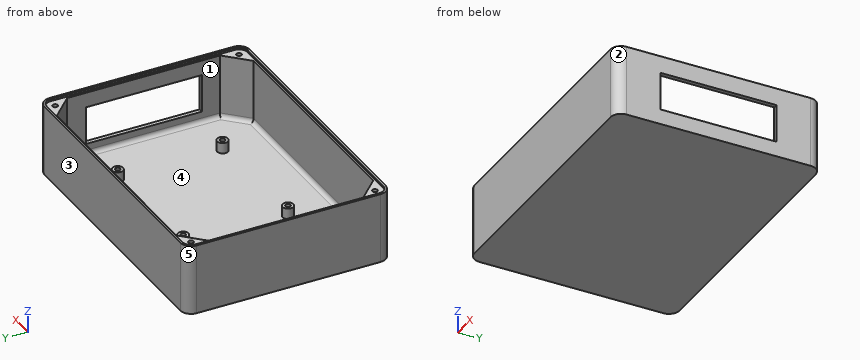
from build123d import *

# Parameters (mm, degrees)
BOSS_EXTRUDE1_DEPTH = 2
BOSS_EXTRUDE2_START = 30
SKETCH2_R           = 3
BOSS_EXTRUDE2_DEPTH = 30
SKETCH3_R           = 1.2
CUT_EXTRUDE1_DEPTH  = 25
BOSS_EXTRUDE3_START = 1
BOSS_EXTRUDE3_DEPTH = 1
SKETCH6_W           = 17.83
SKETCH6_H           = 54.204820934
CUT_EXTRUDE2_DEPTH  = 2
SKETCH7_R           = 2.5
SKETCH7_R_2         = 1.375
SKETCH7_R_3         = 1.2
BOSS_EXTRUDE4_DEPTH = 5
FILLET1_R           = 2


with BuildPart() as part:
    # Sketch1 → Boss-Extrude1 (new body)
    with BuildSketch(Plane(origin=(0, 0, -5), x_dir=(-1, 0, 0), z_dir=(0, 0, -1))):
        with BuildLine():
            Line((77.100439502, -47.051685991), (197.59949644, -47.051685991))
            ThreePointArc((197.59949644, -47.051685991), (201.135030346, -45.587219897), (202.59949644, -42.051685991))
            Line((202.59949644, -42.051685991), (202.59949644, 43.948314009))
            ThreePointArc((202.59949644, 43.948314009), (201.135030346, 47.483847915), (197.59949644, 48.948314009))
            Line((197.59949644, 48.948314009), (77.100439502, 48.948314009))
            ThreePointArc((77.100439502, 48.948314009), (73.564905596, 47.483847915), (72.100439502, 43.948314009))
            Line((72.100439502, 43.948314009), (72.100439502, -42.051685991))
            ThreePointArc((72.100439502, -42.051685991), (73.564905596, -45.587219897), (77.100439502, -47.051685991))
        make_face()
    extrude(amount=BOSS_EXTRUDE1_DEPTH)

    # Sketch2 → Boss-Extrude2 (add)
    # profile 1 of 7: a face of its own
    with BuildSketch(Plane.XY.offset(-5).offset(BOSS_EXTRUDE2_START)):
        with BuildLine():
            ThreePointArc((-202.59949644, -42.051685991), (-201.135030346, -45.587219897), (-197.59949644, -47.051685991))
            Line((-197.59949644, -47.051685991), (-77.100439502, -47.051685991))
            ThreePointArc((-77.100439502, -47.051685991), (-73.564905596, -45.587219897), (-72.100439502, -42.051685991))
            Line((-72.100439502, -42.051685991), (-72.100439502, 43.948314009))
            ThreePointArc((-72.100439502, 43.948314009), (-73.564905596, 47.483847915), (-77.100439502, 48.948314009))
            Line((-77.100439502, 48.948314009), (-197.59949644, 48.948314009))
            ThreePointArc((-197.59949644, 48.948314009), (-201.135030346, 47.483847915), (-202.59949644, 43.948314009))
            Line((-202.59949644, 43.948314009), (-202.59949644, -42.051685991))
        make_face()
        with BuildLine():
            Line((-74.100439502, -34.809045304), (-74.100439502, -42.051685991))
            ThreePointArc((-74.100439502, -42.051685991), (-74.979119158, -44.173006334), (-77.100439502, -45.051685991))
            Line((-77.100439502, -45.051685991), (-84.343080189, -45.051685991))
            Line((-84.343080189, -45.051685991), (-190.356855753, -45.051685991))
            Line((-190.356855753, -45.051685991), (-197.59949644, -45.051685991))
            ThreePointArc((-197.59949644, -45.051685991), (-199.720816783, -44.173006334), (-200.59949644, -42.051685991))
            Line((-200.59949644, -42.051685991), (-200.59949644, -34.809045304))
            Line((-200.59949644, -34.809045304), (-200.59949644, 36.705673322))
            Line((-200.59949644, 36.705673322), (-200.59949644, 43.948314009))
            ThreePointArc((-200.59949644, 43.948314009), (-199.720816783, 46.069634353), (-197.59949644, 46.948314009))
            Line((-197.59949644, 46.948314009), (-190.356855753, 46.948314009))
            Line((-190.356855753, 46.948314009), (-84.343080189, 46.948314009))
            Line((-84.343080189, 46.948314009), (-77.100439502, 46.948314009))
            ThreePointArc((-77.100439502, 46.948314009), (-74.979119158, 46.069634353), (-74.100439502, 43.948314009))
            Line((-74.100439502, 43.948314009), (-74.100439502, 36.705673322))
            Line((-74.100439502, 36.705673322), (-74.100439502, -34.809045304))
        make_face(mode=Mode.SUBTRACT)
    # profile 2 of 7: a face of its own
    with BuildSketch(Plane.XY.offset(-5).offset(BOSS_EXTRUDE2_START)):
        with BuildLine():
            Line((-197.59949644, -45.051685991), (-190.356855753, -45.051685991))
            Line((-190.356855753, -45.051685991), (-200.59949644, -34.809045304))
            Line((-200.59949644, -34.809045304), (-200.59949644, -42.051685991))
            ThreePointArc((-200.59949644, -42.051685991), (-199.720816783, -44.173006334), (-197.59949644, -45.051685991))
        make_face()
    # profile 3 of 7: a face of its own
    with BuildSketch(Plane.XY.offset(-5).offset(BOSS_EXTRUDE2_START)):
        with BuildLine():
            Line((-200.59949644, 36.705673322), (-190.356855753, 46.948314009))
            Line((-190.356855753, 46.948314009), (-197.59949644, 46.948314009))
            ThreePointArc((-197.59949644, 46.948314009), (-199.720816783, 46.069634353), (-200.59949644, 43.948314009))
            Line((-200.59949644, 43.948314009), (-200.59949644, 36.705673322))
        make_face()
    # profile 4 of 7: a face of its own
    with BuildSketch(Plane.XY.offset(-5).offset(BOSS_EXTRUDE2_START)):
        with BuildLine():
            Line((-84.343080189, 46.948314009), (-74.100439502, 36.705673322))
            Line((-74.100439502, 36.705673322), (-74.100439502, 43.948314009))
            ThreePointArc((-74.100439502, 43.948314009), (-74.979119158, 46.069634353), (-77.100439502, 46.948314009))
            Line((-77.100439502, 46.948314009), (-84.343080189, 46.948314009))
        make_face()
    # profile 5 of 7: a face of its own
    with BuildSketch(Plane.XY.offset(-5).offset(BOSS_EXTRUDE2_START)):
        with BuildLine():
            ThreePointArc((-79.221759818, -39.93036562), (-75.952389187, -39.280047401), (-74.100439502, -42.051685991))
            Line((-74.100439502, -42.051685991), (-74.100439502, -34.809045304))
            Line((-74.100439502, -34.809045304), (-79.221759818, -39.93036562))
        make_face()
    # profile 6 of 7: a face of its own
    with BuildSketch(Plane.XY.offset(-5).offset(BOSS_EXTRUDE2_START)):
        with Locations((-77.100439502, -42.051685991)):
            Circle(SKETCH2_R)
    # profile 7 of 7: a face of its own
    with BuildSketch(Plane.XY.offset(-5).offset(BOSS_EXTRUDE2_START)):
        with BuildLine():
            Line((-84.343080189, -45.051685991), (-77.100439502, -45.051685991))
            ThreePointArc((-77.100439502, -45.051685991), (-79.872078107, -43.19973627), (-79.221759818, -39.93036562))
            Line((-79.221759818, -39.93036562), (-84.343080189, -45.051685991))
        make_face()
    extrude(amount=-BOSS_EXTRUDE2_DEPTH)

    # Sketch3 → Cut-Extrude1 (cut)
    with BuildSketch(Plane.XY.offset(25)):
        with Locations((-197.59949644, -42.051685991)):
            Circle(SKETCH3_R)
        with Locations(Location((-77.100439502, -42.051685991, 0), (0, 0, 180))):
            Circle(SKETCH3_R)
        with Locations(Location((-197.59949644, 43.948314009, 0), (0, 0, 180))):
            Circle(SKETCH3_R)
        with Locations((-77.100439502, 43.948314009)):
            Circle(SKETCH3_R)
    extrude(amount=-CUT_EXTRUDE1_DEPTH, mode=Mode.SUBTRACT)

    # Sketch4 → Boss-Extrude3 (add)
    with BuildSketch(Plane.XY.offset(25).offset(BOSS_EXTRUDE3_START)):
        with BuildLine():
            Line((-202.59949644, 43.948314009), (-202.59949644, -42.051685991))
            ThreePointArc((-202.59949644, -42.051685991), (-201.135030346, -45.587219897), (-197.59949644, -47.051685991))
            Line((-197.59949644, -47.051685991), (-77.100439502, -47.051685991))
            ThreePointArc((-77.100439502, -47.051685991), (-73.564905596, -45.587219897), (-72.100439502, -42.051685991))
            Line((-72.100439502, -42.051685991), (-72.100439502, 43.948314009))
            ThreePointArc((-72.100439502, 43.948314009), (-73.564905596, 47.483847915), (-77.100439502, 48.948314009))
            Line((-77.100439502, 48.948314009), (-197.59949644, 48.948314009))
            ThreePointArc((-197.59949644, 48.948314009), (-201.135030346, 47.483847915), (-202.59949644, 43.948314009))
        make_face()
        with BuildLine():
            Line((-201.59949644, 43.948314009), (-201.59949644, -42.051685991))
            ThreePointArc((-201.59949644, -42.051685991), (-200.427923565, -44.880113116), (-197.59949644, -46.051685991))
            Line((-197.59949644, -46.051685991), (-77.100439502, -46.051685991))
            ThreePointArc((-77.100439502, -46.051685991), (-74.272012377, -44.880113116), (-73.100439502, -42.051685991))
            Line((-73.100439502, -42.051685991), (-73.100439502, 43.948314009))
            ThreePointArc((-73.100439502, 43.948314009), (-74.272012377, 46.776741134), (-77.100439502, 47.948314009))
            Line((-77.100439502, 47.948314009), (-197.59949644, 47.948314009))
            ThreePointArc((-197.59949644, 47.948314009), (-200.427923565, 46.776741134), (-201.59949644, 43.948314009))
        make_face(mode=Mode.SUBTRACT)
    extrude(amount=-BOSS_EXTRUDE3_DEPTH)

    # Sketch6 → Cut-Extrude2 (cut)
    with BuildSketch(Plane(origin=(-72.100439502, 0, 0), x_dir=(0, 0, -1), z_dir=(1, 0, 0))):
        with Locations((-9.015, 0.893058013)):
            Rectangle(SKETCH6_W, SKETCH6_H)
    extrude(amount=-CUT_EXTRUDE2_DEPTH, mode=Mode.SUBTRACT)

    # Sketch7 → Boss-Extrude4 (add)
    # profile 1 of 8: a face of its own
    with BuildSketch(Plane.XY.offset(-5)):
        with Locations(Location((-155.600439502, -23.551685991, 0), (0, 0, 180))):
            Circle(SKETCH7_R)
        with Locations((-155.600439502, -23.551685991)):
            Circle(SKETCH7_R_2, mode=Mode.SUBTRACT)
    # profile 2 of 8: a face of its own
    with BuildSketch(Plane.XY.offset(-5)):
        with Locations((-155.600439502, -23.551685991)):
            Circle(SKETCH7_R_2)
        with Locations((-155.600439502, -23.551685991)):
            Circle(SKETCH7_R_3, mode=Mode.SUBTRACT)
    # profile 3 of 8: a face of its own
    with BuildSketch(Plane.XY.offset(-5)):
        with Locations(Location((-155.600439502, 25.448314009, 0), (0, 0, 180))):
            Circle(SKETCH7_R)
        with Locations((-155.600439502, 25.448314009)):
            Circle(SKETCH7_R_2, mode=Mode.SUBTRACT)
    # profile 4 of 8: a face of its own
    with BuildSketch(Plane.XY.offset(-5)):
        with Locations((-155.600439502, 25.448314009)):
            Circle(SKETCH7_R_2)
        with Locations((-155.600439502, 25.448314009)):
            Circle(SKETCH7_R_3, mode=Mode.SUBTRACT)
    # profile 5 of 8: a face of its own
    with BuildSketch(Plane.XY.offset(-5)):
        with Locations(Location((-97.600439502, 25.448314009, 0), (0, 0, 180))):
            Circle(SKETCH7_R)
        with Locations((-97.600439502, 25.448314009)):
            Circle(SKETCH7_R_2, mode=Mode.SUBTRACT)
    # profile 6 of 8: a face of its own
    with BuildSketch(Plane.XY.offset(-5)):
        with Locations((-97.600439502, 25.448314009)):
            Circle(SKETCH7_R_2)
        with Locations((-97.600439502, 25.448314009)):
            Circle(SKETCH7_R_3, mode=Mode.SUBTRACT)
    # profile 7 of 8: a face of its own
    with BuildSketch(Plane.XY.offset(-5)):
        with Locations(Location((-97.600439502, -23.551685991, 0), (0, 0, 180))):
            Circle(SKETCH7_R)
        with Locations((-97.600439502, -23.551685991)):
            Circle(SKETCH7_R_2, mode=Mode.SUBTRACT)
    # profile 8 of 8: a face of its own
    with BuildSketch(Plane.XY.offset(-5)):
        with Locations((-97.600439502, -23.551685991)):
            Circle(SKETCH7_R_2)
        with Locations((-97.600439502, -23.551685991)):
            Circle(SKETCH7_R_3, mode=Mode.SUBTRACT)
    extrude(amount=BOSS_EXTRUDE4_DEPTH)

    # Fillet1
    fillet1_edges = [part.edges().sort_by_distance(p)[0] for p in [
        (-79.221759845, -39.930365647, -5),
        (-195.478176096, 41.826993666, -5),
        (-74.100439502, 0.948314009, -5),
        (-79.221759845, 41.826993666, -5),
        (-137.349967971, 46.948314009, -5),
        (-200.59949644, 0.948314009, -5),
        (-195.478176096, -39.930365647, -5),
        (-137.349967971, -45.051685991, -5),
    ]]
    fillet(fillet1_edges, radius=FILLET1_R)


solid = part.part
Check sheet for the modelled part. Datum: model origin and axes. Units: mm. Face numbers are marked on the shaded views. A direction names the side the tool comes from. Coordinates: 2 decimals unless noted, no trailing zeros. Loops run counter-clockwise (first coordinate to the right, second up) from the corner with the lowest first, then second, coordinate; pieces in that order, holes last. Notation, with made-up numbers: (-10, 63.5) -> (35, 63.5) arc R9 cw to (35, 80.5) -> close; hole circle Ø6 at (55.5, 49.25). An arc over 180 degrees is marked (long way). Write item = value, one per line. Start each with the question number.
1. Depth check by flat-ended pin: P1, Ø6, axis at x = -189, y = -35.5, coming from the +Z side; P2, Ø1, axis at y = -3, z = 2.5, coming from the +X side; P3, Ø3, axis at x = -197.6, y = 43.95, coming from the +Z side. Enter the tip coordinate at first touch or a pass-through.
2. Section check A-A on z = 9. Record the cut outline in (x, y), then the cut area to 3 significant figures.
3. Draft check along Y on the marked faces 1, 2 and 3. Enter one of: released by +Y, released by -Y, zero draft, split by the parting line, or undercut.
4. Material ranges on line 1 (Y direction, x = -89, z = 12); line 2 (X direction, y = 31, z = 12); line 3 (X direction, y = 24, z = -1), recorded low to high.
5. Section check D-D on x = -187. Record the cut outline in (y, z), then the cut area to 3 significant figures.
6. Section check C-C on z = 21. Record the cut outline in (x, y), then the cut area to 3 significant figures.
7. Tool access check on the marked faces 4 and 5. Record the directions out of +Z, -Z, +X, -X, +Y, -Y that give a thin tool (end or side, any length) a straight path to the whole face; none if there is none.
8. Section check B-B on y = 19.5. Record the cut outline in (x, z).
Responses:
q1.P1 = -5
q1.P2 = -200.6
q1.P3 = 25
q2.outline = (-202.6, -42.05) arc R5 ccw to (-197.6, -47.05) -> (-77.1, -47.05) arc R5 ccw to (-72.1, -42.05) -> (-72.1, -26.21) -> (-74.1, -26.21) -> (-74.1, -34.81) -> (-84.34, -45.05) -> (-190.36, -45.05) -> (-200.6, -34.81) -> (-200.6, 36.71) -> (-190.36, 46.95) -> (-84.34, 46.95) -> (-74.1, 36.71) -> (-74.1, 28) -> (-72.1, 28) -> (-72.1, 43.95) arc R5 ccw to (-77.1, 48.95) -> (-197.6, 48.95) arc R5 ccw to (-202.6, 43.95) -> close; hole circle Ø2.4 at (-197.6, -42.05); hole circle Ø2.4 at (-197.6, 43.95); hole circle Ø2.4 at (-77.1, -42.05); hole circle Ø2.4 at (-77.1, 43.95)
q2.area = 952 mm2
q3.face_1 = undercut
q3.face_2 = released by -Y
q3.face_3 = released by +Y
q4.line_1 = -47.05 to -45.05, 46.95 to 48.95
q4.line_2 = -202.6 to -200.6, -74.1 to -72.1
q4.line_3 = -202.6 to -200.6, -157.64 to -153.56, -99.64 to -95.56, -74.1 to -72.1
q5.outline = (-47.05, -7) -> (48.95, -7) -> (48.95, 26) -> (47.95, 26) -> (47.95, 25) -> (46.95, 25) -> (46.95, -3) arc R2 cw to (44.95, -5) -> (-43.05, -5) arc R2 cw to (-45.05, -3) -> (-45.05, 25) -> (-46.05, 25) -> (-46.05, 26) -> (-47.05, 26) -> close
q5.area = 316 mm2
q6.outline = (-202.6, -42.05) arc R5 ccw to (-197.6, -47.05) -> (-77.1, -47.05) arc R5 ccw to (-72.1, -42.05) -> (-72.1, 43.95) arc R5 ccw to (-77.1, 48.95) -> (-197.6, 48.95) arc R5 ccw to (-202.6, 43.95) -> close; hole (-200.6, -34.81) -> (-190.36, -45.05) -> (-84.34, -45.05) -> (-74.1, -34.81) -> (-74.1, 36.71) -> (-84.34, 46.95) -> (-190.36, 46.95) -> (-200.6, 36.71) -> close; hole circle Ø2.4 at (-197.6, -42.05); hole circle Ø2.4 at (-197.6, 43.95); hole circle Ø2.4 at (-77.1, -42.05); hole circle Ø2.4 at (-77.1, 43.95)
q6.area = 1,060 mm2
q7.face_4 = +Z
q7.face_5 = +Z, -Z, -X, +Y
q8.outline = (-202.6, -7) -> (-72.1, -7) -> (-72.1, 0.1) -> (-74.1, 0.1) -> (-74.1, -3) arc R2 cw to (-76.1, -5) -> (-198.6, -5) arc R2 cw to (-200.6, -3) -> (-200.6, 25) -> (-201.6, 25) -> (-201.6, 26) -> (-202.6, 26) -> close; (-74.1, 17.93) -> (-72.1, 17.93) -> (-72.1, 26) -> (-73.1, 26) -> (-73.1, 25) -> (-74.1, 25) -> close
